from build123d import *

# Parameters (mm, degrees)
F0_W      = 2000
F0_H      = 32
F1_DEPTH  = 200
F2_SIZE   = 12
F3_SIZE   = 5
F5_DEPTH  = 32
F6_SIZE   = 4.99999
F7_SIZE   = 4.99999
F9_DEPTH  = 2097
F10_SIZE2 = 15
F10_SIZE  = 20


# Not quite as in the source:
# - a fillet or chamfer is up to 0.001 mm smaller than in the source, because OpenCascade refuses the exact size


with BuildPart() as f1:
    # F0 (on Front) → F1 (new body)
    with BuildSketch(Plane.XZ):
        with Locations((-1000, 16)):
            Rectangle(F0_W, F0_H)
    extrude(amount=F1_DEPTH)

    # F2
    f2_edges = [f1.edges().sort_by_distance(p)[0] for p in [
        (-1000, 0, 32),
    ]]
    chamfer(f2_edges, length=F2_SIZE)

    # F3
    f3_edges = [f1.edges().sort_by_distance(p)[0] for p in [
        (-1000, -200, 32),
    ]]
    chamfer(f3_edges, length=F3_SIZE)

    # F4 (on Top) → F5 (join)
    with BuildSketch(Plane.XY):
        Polygon((30, -200), (0, 0), (0, -200), align=None)
        Polygon((-2000, 0), (-2030, -200), (-2000, -200), align=None)
    extrude(amount=F5_DEPTH)

    # F6 (size 5 in the source; OpenCascade refuses exactly that, so slightly less here)
    f6_edges = [f1.edges().sort_by_distance(p)[0] for p in [
        (-2015, -200, 32),
    ]]
    chamfer(f6_edges, length=F6_SIZE)

    # F7 (size 5 in the source; OpenCascade refuses exactly that, so slightly less here)
    f7_edges = [f1.edges().sort_by_distance(p)[0] for p in [
        (15, -200, 32),
    ]]
    chamfer(f7_edges, length=F7_SIZE)

    # F8 (on Right) → F9 (cut, symmetric)
    with BuildSketch(Plane.YZ):
        Polygon((-12, 32), (0, 20), (0, 32), align=None)
    extrude(amount=F9_DEPTH, both=True, mode=Mode.SUBTRACT)

    # F10
    f10_edges = [f1.edges().sort_by_distance(p)[0] for p in [
        (-1000, -200, 0),
        (-2015, -100, 0),
        (15, -100, 0),
    ]]
    f10_side = f1.faces().sort_by_distance((-1000, -100.492611, 0))[0]
    chamfer(f10_edges, length=F10_SIZE, length2=F10_SIZE2, reference=f10_side)


solid = f1.part
Input: part model. Units: mm. Frame: model coordinates. Round coordinates to 2 decimals unless told otherwise and drop trailing zeros. Write each loop counter-clockwise with the first axis right and the second up, starting at its lowest first coordinate (ties: lowest second). Pieces come first, ordered by that corner, then holes.
1) Cut plane A-A (x = -1673). Return the cut outline in (y, z), then the cut area to 3 significant figures.
2) Contact query for flat-ended pins moving along their axis: P1, Ø3, axis at y = -55.5, z = 12, coming from the +X side; P2, Ø3, axis at x = -1468.5, z = 6.5, coming from the -Y side; P3, Ø5.5, axis at y = -198, z = 29.5, coming from the -X side. Output: stop coordinate, or through.
3) Cut plane B-B (y = -40.5). Return the cut outline in (x, z) (3 decimals).
4) Ray query, L1, parallel to X at y = -42.5, z = 19.5 (3 decimals); L2, parallel to X at y = -182, z = 22; L3, parallel to Z at x = -236, y = -9. Return the intervals inside material, ascending.
5) Cut plane C-C (z = 8.5). Return the cut outline in (x, y), then the cut area to 3 significant figures.
Geometry says:
1. outline: (-200, 15) - (-180, 0) - (0, 0) - (0, 20) - (-12, 32) - (-195, 32) - (-200, 27) - close
1. area: 6,170 mm2
2. P1: stops at x = 6.32
2. P2: stops at y = -190.67
2. P3: stops at x = -2029.95
3. outline: (-2006.075, 15) - (-1985.851, 0) - (-14.149, 0) - (6.075, 15) - (6.075, 32) - (-2006.075, 32) - close
4. L1: x = -2006.375 to 6.375
4. L2: x = -2027.3 to 27.3
4. L3: z = 0 to 29
5. outline: (-2019.94, -191.33) - (19.94, -191.33) - (-8.76, 0) - (-1991.24, 0) - close
5. area: 385,000 mm2
